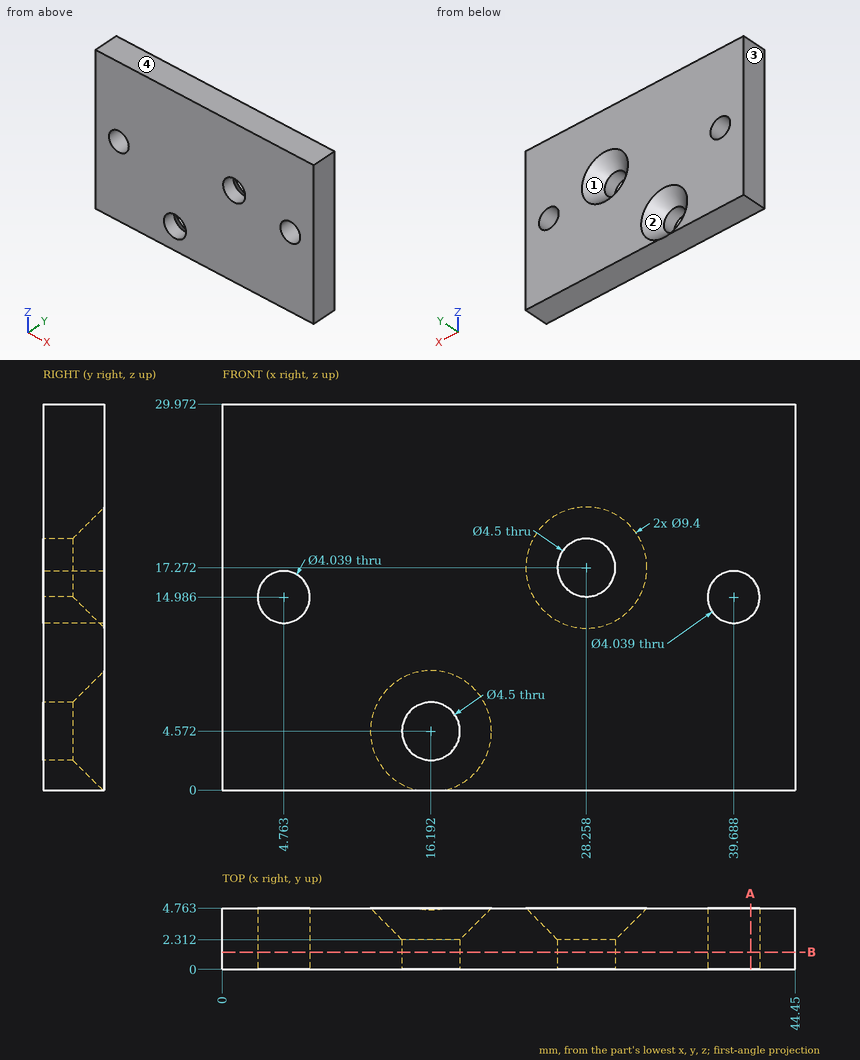
Print and shaded views of the part. All mm, measured from the part's lowest x, y and z. Give positions to 0.01 mm unless a question says otherwise; leave off trailing zeros. Loops run counter-clockwise (first coordinate to the right, second up) from the corner with the lowest first, then second, coordinate; pieces in that order, holes last.
1) Flat gauge pins, fed straight in: pin 1 Ø2.5 at (x, z) = (28.26, 17.27) entering from +Y; pin 2 Ø5 at (x, z) = (16.19, 4.57) entering from +Y (1 decimal). Where does each tip first touch, or does it go through?
2) Saw through at A-A (x = 41). Write the cut outline in (y, z).
3) Wall check: line 1 (Z direction, x = 3, y = 3.6) (1 decimal); line 2 (Z direction, x = 4, y = 1.8) (1 decimal). Give the ranges that are in metal, low to high.
4) Pull direction X, two halves, no side cores. Call the marked faces 1, 2, 3 and 4: +X half, -X half, draft (parallel to the pull), parting line (faces both ways), or undercut.
5) Saw through at B-B (y = 1.35). Count the separate pieces of the cut face and the enclosed holes in it, plus the area to 4 significant figures.
Answer block:
1. pin 1: passes through
1. pin 2: stops at y = 2.6
2. outline: (0, 0) - (4.76, 0) - (4.76, 13.45) - (0, 13.45) - close; (0, 16.52) - (4.76, 16.52) - (4.76, 29.97) - (0, 29.97) - close
3. line 1: z = 0 to 14, 16 to 30
3. line 2: z = 0 to 13.1, 16.9 to 30
4. face 1: undercut
4. face 2: undercut
4. face 3: -X half
4. face 4: draft
5. separate pieces: 1
5. enclosed holes: 4
5. area: 1,275 mm2
